from build123d import *

# Parameters (mm, degrees)
SM_BASE_FLANGE_1_DEPTH = 22.5
SKETCH_3_R             = 19
CUT_EXTRUDE_1_DEPTH    = 71.75485849
FILLET_1_R             = 10
SKETCH_6_R             = 3
CUT_EXTRUDE_3_DEPTH    = 70.06699646


# Sheet-metal steps are written as plain solids
with BuildPart() as part:
    # Sketch 1 → 基体-法兰1 (new, symmetric)
    with BuildSketch(Plane.XY):
        with BuildLine():
            Line((-60, 0), (-2.7366, 0))
            ThreePointArc((-2.7366, 0), (-0.801531583, -0.801531583), (0, -2.7366))
            Line((0, -2.7366), (0, -30))
            Line((0, -30), (-2, -30))
            Line((-2, -30), (-2, -2.7366))
            ThreePointArc((-2, -2.7366), (-2.215745145, -2.215745145), (-2.7366, -2))
            Line((-2.7366, -2), (-60, -2))
            Line((-60, -2), (-60, 0))
        make_face()
    extrude(amount=SM_BASE_FLANGE_1_DEPTH, both=True)

    # 草图3 → 切除-拉伸1 (cut, through all)
    with BuildSketch(Plane(origin=(0, 0, 0), x_dir=(1, 0, 0), z_dir=(0, 1, 0))):
        with Locations(Location((-35, 0, 0), (0, 0, 270))):
            Circle(SKETCH_3_R)
    extrude(amount=-CUT_EXTRUDE_1_DEPTH, mode=Mode.SUBTRACT)

    # 圆角1
    fillet_1_edges = [part.edges().sort_by_distance(p)[0] for p in [
        (-60, -1, 22.5),
        (-1, -30, 22.5),
        (-60, -1, -22.5),
        (-1, -30, -22.5),
    ]]
    fillet(fillet_1_edges, radius=FILLET_1_R)

    # 草图6 → 切除-拉伸3 (cut, through all)
    with BuildSketch(Plane.ZY.offset(2)):
        with Locations(Location((11, -24, 0), (0, 0, 270))):
            Circle(SKETCH_6_R)
        with Locations(Location((-8.052558883, -13, 0), (0, 0, 270))):
            Circle(SKETCH_6_R)
    extrude(amount=-CUT_EXTRUDE_3_DEPTH, mode=Mode.SUBTRACT)


solid = part.part
Check sheet for the modelled part. Datum: model origin and axes. Units: mm. A direction names the side the tool comes from. Round coordinates to 2 decimals unless told otherwise and drop trailing zeros. Loops run counter-clockwise (first coordinate to the right, second up) from the corner with the lowest first, then second, coordinate; pieces in that order, holes last. Notation, with made-up numbers: (83.25, -2) - (103.25, -2) arc R18 cw to (103.25, 11) - close; hole circle Ø6 at (-36.5, 32.25). An arc over 180 degrees is marked (long way). Answer as CSV lines item,"result". Start each with the question number.
Item 1: Section check D-D (z = 9). Record the boundary of the cut face in (x, y).
Item 2: Section check C-C (y = -13). Record the boundary of the cut face in (x, z).
Item 3: Depth check by flat-ended pin: P1, Ø3, axis at x = -13, z = -1, coming from the -Y side; P2, Ø1, axis at y = -25.5, z = 15.5, coming from the -X side. Enter the tip coordinate at first touch or a pass-through.
Item 4: Section check B-B (x = -35). Record the boundary of the cut face in (y, z).
Item 5: Scan lines: line 1 (Z direction, x = -1.1, y = -13); line 2 (Y direction, x = -13, z = 16). Record each from-to range of solid material in increasing order. Write a range as [from, to].
Item 6: Section check A-A (z = 0). Record the boundary of the cut face in (x, y), and give its area (3 significant figures).
Item 7: Release check for a two-part mould opening along Y. For faces 1 (the flat face through (0, -16, 0)), 2 (the cylindrical face through (-1, -21, 11)), 3 (the cylindrical face through (-1.01, -10.62, -9.88)), 4 (the flat face through (-1, -30, 0)) record: +Y half, -Y half, draft (parallel to the pull), parting line (faces both ways), or undercut.
Item 8: Set-up check for faces 5 (the flat face through (-2, -17, 0)), 6 (the flat face through (-19.3, -1.8, -22.5)): record each of +Z, -Z, +X, -X, +Y, -Y from which the full face is reachable in a straight line by a thin tool's end or side.
Report:
1,outline,"(-60, -2) - (-51.73, -2) - (-51.73, 0) - (-60, 0) - close; (-18.27, -2) - (-2.74, -2) arc R0.74 cw to (-2, -2.74) - (-2, -21.76) - (0, -21.76) - (0, -2.74) arc R2.74 ccw to (-2.74, 0) - (-18.27, 0) - close; (-2, -30) - (0, -30) - (0, -26.24) - (-2, -26.24) - close"
2,outline,"(-2, -22.5) - (0, -22.5) - (0, -11.05) - (-2, -11.05) - close; (-2, -5.05) - (0, -5.05) - (0, 22.5) - (-2, 22.5) - close"
3,P1,"stops at y = -2"
3,P2,"stops at x = -2"
4,outline,"(-2, -22.5) - (0, -22.5) - (0, -19) - (-2, -19) - close; (-2, 19) - (0, 19) - (0, 22.5) - (-2, 22.5) - close"
5,line 1,"z = [-22.5, -11.05], [-5.05, 22.5]"
5,line 2,"y = [-2, 0]"
6,outline,"(-60, -2) - (-54, -2) - (-54, 0) - (-60, 0) - close; (-16, -2) - (-2.74, -2) arc R0.74 cw to (-2, -2.74) - (-2, -30) - (0, -30) - (0, -2.74) arc R2.74 ccw to (-2.74, 0) - (-16, 0) - close"
6,area,"98.5 mm2"
7,face 1,"draft"
7,face 2,"undercut"
7,face 3,"undercut"
7,face 4,"-Y half"
8,face 5,"+Z, -Z, -X, -Y"
8,face 6,"-Z, +X, -X, +Y, -Y"
